Can you work these out from the model? Positions are in its coordinate system, mm. A direction names the side the tool comes from. Give positions to 0.01 mm unless a question says otherwise; leave off trailing zeros. Order: outer loops, then holes, each group sorted by start corner. A loop starts at its lowest first (then second) coordinate and runs counter-clockwise, first axis right, second up.
Item 1: I want a section at A-A, the plane x = -96.5. Write out the boundary of the cut face in (y, z) (3 decimals).
Item 2: I want a section at C-C, the plane x = 0. Count the separate pieces of the cut face and the enclosed holes in it, then the cut area to 3 significant figures.
Item 3: If we mould it in two halves opening along X, with no side actions, what happens to faces 1 (the cylindrical face through (-117.64, 0.9, 6.08)), 2 (the flat face through (-116, 1, 12)), 3 (the cylindrical face through (123.997, 39.048, 5.916))? For each: +X half, -X half, draft (parallel to the pull), parting line (faces both ways), or undercut.
Item 4: I want a section at D-D, the plane y = 26. Write out the boundary of the cut face in (x, z), then the cut area to 3 significant figures.
Item 5: Which directions (+Z, -Z, +X, -X, +Y, -Y) give clear straight access to the entire face, cutting with the end or side of a thin tool? Please do faces 4 (the flat face through (-88, 56, 7)), 5 (the cylindrical face through (-22.112, -99.574, 5.423)).
Item 6: I want a section at B-B, the plane y = -120.5. Write out the boundary of the cut face in (x, z), then the cut area to 3 significant figures.
Item 7: If I drill on line 1 along Y through (x, z) = (0, 6.5); line 2 along Y through (x, z) = (0, 8.2); line 3 along Y through (x, z) = (0, 11.2), over which ranges is the centre line in solid material (lowest first)?
Item 8: I'm going to push flat-ended pins straight in: pin 1 Ø8 at (x, y) = (85.21, 85.21) entering from +Z; pin 2 Ø12 at (y, z) = (56.5, 17) entering from +X; pin 3 Ø8 at (x, z) = (37.5, 5) entering from +Y. Where does each tip first touch, or does it pass through?
```python
from build123d import *

# Parameters (mm, degrees)
F0_R      = 130
F0_R_2    = 102
F1_DEPTH  = 12
F2_R      = 115.5
F2_R_2    = 110.5
F3_DEPTH  = 2.5
F4_R      = 107
F4_R_2    = 104
F5_DEPTH  = 5
F6_R      = 104
F6_R_2    = 102
F7_DEPTH  = 1
F8_R      = 3
F9_DEPTH  = 12
F10_DEPTH = 10
F11_SIZE  = 1
F12_SIZE  = 1


with BuildPart() as f1:
    # F0 (on Top) → F1 (new body)
    with BuildSketch(Plane.XY):
        Circle(F0_R)
        Circle(F0_R_2, mode=Mode.SUBTRACT)
    extrude(amount=F1_DEPTH)

    # F2 (on face) → F3 (cut)
    with BuildSketch(Plane.XY.offset(12)):
        Circle(F2_R)
        Circle(F2_R_2, mode=Mode.SUBTRACT)
    extrude(amount=-F3_DEPTH, mode=Mode.SUBTRACT)

    # F4 (on face) → F5 (cut)
    with BuildSketch(Plane.XY.offset(12)):
        Circle(F4_R)
        Circle(F4_R_2, mode=Mode.SUBTRACT)
    extrude(amount=-F5_DEPTH, mode=Mode.SUBTRACT)

    # F6 (on face) → F7 (cut)
    with BuildSketch(Plane.XY.offset(12)):
        Circle(F6_R)
        Circle(F6_R_2, mode=Mode.SUBTRACT)
    extrude(amount=-F7_DEPTH, mode=Mode.SUBTRACT)

    # F8 (on face) → F9 (cut)
    with BuildSketch(Plane.XY.offset(12)):
        with Locations((-120.5, 0)):
            Circle(F8_R)
        with Locations((-85.206367, 85.206367)):
            Circle(F8_R)
        with Locations((0, 120.5)):
            Circle(F8_R)
        with Locations((120.5, 0)):
            Circle(F8_R)
        with Locations((85.206367, 85.206367)):
            Circle(F8_R)
        with Locations((85.206367, -85.206367)):
            Circle(F8_R)
        with Locations((0, -120.5)):
            Circle(F8_R)
        with Locations((-85.206367, -85.206367)):
            Circle(F8_R)
    extrude(amount=-F9_DEPTH, mode=Mode.SUBTRACT)

    # F8 (on face) → F10 (join)
    with BuildSketch(Plane.XY.offset(12)):
        with Locations((-46.113354, 111.327484)):
            Circle(F8_R)
        with Locations((-46.113354, -111.327484)):
            Circle(F8_R)
    extrude(amount=F10_DEPTH)

    # F11
    f11_edges = [f1.edges().sort_by_distance(p)[0] for p in [
        (-49.113354, -111.327484, 22),
    ]]
    chamfer(f11_edges, length=F11_SIZE)

    # F12
    f12_edges = [f1.edges().sort_by_distance(p)[0] for p in [
        (-49.113354, 111.327484, 22),
    ]]
    chamfer(f12_edges, length=F12_SIZE)


solid = f1.part
```
Results list:
1. outline: (-87.108, 0) - (-33.042, 0) - (-33.042, 11) - (-38.778, 11) - (-38.778, 7) - (-46.225, 7) - (-46.225, 12) - (-53.833, 12) - (-53.833, 9.5) - (-63.467, 9.5) - (-63.467, 12) - (-87.108, 12) - close; (33.042, 0) - (87.108, 0) - (87.108, 12) - (63.467, 12) - (63.467, 9.5) - (53.833, 9.5) - (53.833, 12) - (46.225, 12) - (46.225, 7) - (38.778, 7) - (38.778, 11) - (33.042, 11) - close
2. separate pieces: 4
2. enclosed holes: 0
2. area: 469 mm2
3. face 1: undercut
3. face 2: draft
3. face 3: parting line
4. outline: (-127.37, 0) - (-98.63, 0) - (-98.63, 11) - (-100.7, 11) - (-100.7, 7) - (-103.79, 7) - (-103.79, 12) - (-107.4, 12) - (-107.4, 9.5) - (-112.54, 9.5) - (-112.54, 12) - (-127.37, 12) - close; (98.63, 0) - (127.37, 0) - (127.37, 12) - (112.54, 12) - (112.54, 9.5) - (107.4, 9.5) - (107.4, 12) - (103.79, 12) - (103.79, 7) - (100.7, 7) - (100.7, 11) - (98.63, 11) - close
4. area: 629 mm2
5. face 4: +Z
5. face 5: +Z, -Z
6. outline: (-48.78, 0) - (-3, 0) - (-3, 12) - (-48.78, 12) - close; (3, 0) - (48.78, 0) - (48.78, 12) - (3, 12) - close
6. area: 1,100 mm2
7. line 1: y = -130 to -123.5, -117.5 to -102, 102 to 117.5, 123.5 to 130
7. line 2: y = -130 to -123.5, -117.5 to -107, -104 to -102, 102 to 104, 107 to 117.5, 123.5 to 130
7. line 3: y = -130 to -123.5, -117.5 to -115.5, -110.5 to -107, 107 to 110.5, 115.5 to 117.5, 123.5 to 130
8. pin 1: stops at z = 12
8. pin 2: stops at x = 118.62
8. pin 3: stops at y = 125.61
